Here's how the part is built. I have some questions about the finished solid (model axes, mm). A direction names the side the tool comes from. Round coordinates to 2 decimals unless told otherwise and drop trailing zeros. Order: outer loops, then holes, each group sorted by start corner. A loop starts at its lowest first (then second) coordinate and runs counter-clockwise, first axis right, second up. Notation, with made-up numbers: (5.25, 16.25) - (44.25, 16.25) arc R15 ccw to (44.25, 38.25) - close; hole circle Ø10 at (19.25, 43.5). An arc over 180 degrees is marked (long way). Answer as a JSON object with one key per item and string values.
```python
from build123d import *

# Parameters (mm, degrees)
SKETCH_R           = 8.5
SKETCH_R_2         = 1.5
PAD_DEPTH          = 3
SKETCH001_R        = 2
SKETCH001_R_2      = 0.5
POCKET_DEPTH       = 3
POLARPATTERN_COUNT = 4
SKETCH002_R        = 2
PAD001_DEPTH       = 3


with BuildPart() as part:
    # Sketch → Pad (new body)
    with BuildSketch(Plane.XY):
        Circle(SKETCH_R)
        Circle(SKETCH_R_2, mode=Mode.SUBTRACT)
    extrude(amount=PAD_DEPTH)

    # Sketch001 → Pocket (cut)
    with BuildSketch(Plane(origin=(0, 0, 0), x_dir=(1, 0, 0), z_dir=(0, 0, -1))):
        with Locations((0, 6)):
            Circle(SKETCH001_R)
        with Locations((4.24264, 4.24264)):
            Circle(SKETCH001_R_2)
    pocket = extrude(amount=-POCKET_DEPTH, mode=Mode.SUBTRACT)

    # PolarPattern: Pocket ×4 about axis
    polarpattern_axis = Axis((0, 0, 0), (0, 0, -1))
    for i in range(1, POLARPATTERN_COUNT):
        add(pocket.rotate(polarpattern_axis, i * 360 / POLARPATTERN_COUNT), mode=Mode.SUBTRACT)

    # Sketch002 → Pad001 (new body)
    with BuildSketch(Plane(origin=(0, 0, 0), x_dir=(1, 0, 0), z_dir=(0, 0, -1))):
        Circle(SKETCH002_R)
    extrude(amount=PAD001_DEPTH)


solid = part.part
```
1. For P1, Ø0.9, axis at x = -0.5, y = 0, coming from the +Z side; P2, Ø3, axis at x = 2.5, z = 2.5, coming from the +Y side; P3, Ø1, axis at x = -3.5, z = 1.5, coming from the +Y side, each with a flat end and sliding along its axis, tell me the tip position at first contact or that it passes through.
Responses:
{"P1": "z = 0", "P2": "y = 8.44", "P3": "y = 7.95"}
2. Thinking about a two-plate mould opening in Y: for faces 1 (the face through (4.57, 7.167, 1.479)), 2 (the face through (0, 0, -3)), 3 (the face through (-4.18, 4.74, 1.48)), which applies, pulls with the +Y half, pulls with the -Y half, needs draft (parallel to the pull), parting line crosses it, or undercut?
Responses:
{"face 1": "parting line crosses it", "face 2": "needs draft", "face 3": "undercut"}
3. If I drill on L1, parallel to X at y = -1.75, z = 0.15; L2, parallel to Z at x = -5, y = 5.5; L3, parallel to X at y = -6, z = 1.95, over which ranges is the centre line in solid material (lowest first)? Write a range as [from, to].
Responses:
{"L1": "[-8.32, -6.97], [-5.03, 5.03], [6.97, 8.32]", "L2": "[0, 3]", "L3": "[-6.02, -2], [2, 6.02]"}
4. Imagine slicing it at B-B (y = 6). List the corners of the cut face in (x, z) for me.
Responses:
{"outline": "(-6.02, 0) - (-2, 0) - (-2, 3) - (-6.02, 3) - close; (2, 0) - (6.02, 0) - (6.02, 3) - (2, 3) - close"}
5. For faces 4 (the face through (-1.5, 0.07, 1.48)), 5 (the face through (0, 2, -1)), 6 (the face through (0, -8, 1)), which set-ups out of +Z, -Z, +X, -X, +Y, -Y let a thin tool reach every point of the face, with its end or its side?
Responses:
{"face 4": "+Z", "face 5": "-Z", "face 6": "+Z, -Z"}
6. Imagine slicing it at A-A (x = 0). List the corners of the cut face in (y, z) for me, plus the area to 3 significant figures.
Responses:
{"outline": "(-8.5, 0) - (-8, 0) - (-8, 3) - (-8.5, 3) - close; (-4, 0) - (-2, 0) - (-2, -3) - (2, -3) - (2, 0) - (4, 0) - (4, 3) - (1.5, 3) - (1.5, 0) - (-1.5, 0) - (-1.5, 3) - (-4, 3) - close; (8, 0) - (8.5, 0) - (8.5, 3) - (8, 3) - close", "area": "30.0 mm2"}
